CAD build for the part. Positions are in the model's coordinates, mm. Give positions to 0.01 mm unless a question says otherwise; leave off trailing zeros. Write each loop counter-clockwise with the first axis right and the second up, starting at its lowest first coordinate (ties: lowest second). Pieces come first, ordered by that corner, then holes. Notation, with made-up numbers: (-3.75, 54) -> (41.25, 54) arc R13 cw to (41.25, 71) -> close; hole circle Ø11 at (20.25, 67). An arc over 180 degrees is marked (long way). Answer in a Markdown table with one row per item. Add a question column.
```python
from build123d import *

# Parameters (mm, degrees)
SKETCH1_W           = 809.625
SKETCH1_H           = 555.625
SKETCH1_R           = 1.27
SKETCH1_W_2         = 136.525
SKETCH1_H_2         = 184.76057441
BOSS_EXTRUDE1_DEPTH = 4.318
CUT_EXTRUDE2_DEPTH  = 5.318


with BuildPart() as part:
    # Sketch1 → Boss-Extrude1 (new body, symmetric)
    with BuildSketch(Plane.XY):
        Rectangle(SKETCH1_W, SKETCH1_H)
        with Locations((319.0875, 265.1125)):
            Circle(SKETCH1_R, mode=Mode.SUBTRACT)
        with Locations((344.4875, 265.1125)):
            Circle(SKETCH1_R, mode=Mode.SUBTRACT)
        with Locations((369.8875, 265.1125)):
            Circle(SKETCH1_R, mode=Mode.SUBTRACT)
        with Locations((392.1125, 217.4875)):
            Circle(SKETCH1_R, mode=Mode.SUBTRACT)
        with Locations((392.1125, 242.8875)):
            Circle(SKETCH1_R, mode=Mode.SUBTRACT)
        with Locations((392.1125, 268.2875)):
            Circle(SKETCH1_R, mode=Mode.SUBTRACT)
        with Locations((-315.9125, -265.1125)):
            Circle(SKETCH1_R, mode=Mode.SUBTRACT)
        with Locations((-341.3125, -265.1125)):
            Circle(SKETCH1_R, mode=Mode.SUBTRACT)
        with Locations((-366.7125, -265.1125)):
            Circle(SKETCH1_R, mode=Mode.SUBTRACT)
        with Locations((-392.1125, -214.3125)):
            Circle(SKETCH1_R, mode=Mode.SUBTRACT)
        with Locations((-392.1125, -239.7125)):
            Circle(SKETCH1_R, mode=Mode.SUBTRACT)
        with Locations((-392.1125, -265.1125)):
            Circle(SKETCH1_R, mode=Mode.SUBTRACT)
        with Locations((-315.9125, 265.1125)):
            Circle(SKETCH1_R, mode=Mode.SUBTRACT)
        with Locations((-341.3125, 265.1125)):
            Circle(SKETCH1_R, mode=Mode.SUBTRACT)
        with Locations((-366.7125, 265.1125)):
            Circle(SKETCH1_R, mode=Mode.SUBTRACT)
        with Locations((-392.1125, 217.4875)):
            Circle(SKETCH1_R, mode=Mode.SUBTRACT)
        with Locations((-392.1125, 242.8875)):
            Circle(SKETCH1_R, mode=Mode.SUBTRACT)
        with Locations((-392.1125, 268.2875)):
            Circle(SKETCH1_R, mode=Mode.SUBTRACT)
        with Locations((319.0875, -265.1125)):
            Circle(SKETCH1_R, mode=Mode.SUBTRACT)
        with Locations((392.1125, -188.9125)):
            Circle(SKETCH1_R, mode=Mode.SUBTRACT)
        with Locations((392.1125, -214.3125)):
            Circle(SKETCH1_R, mode=Mode.SUBTRACT)
        with Locations((392.1125, -239.7125)):
            Circle(SKETCH1_R, mode=Mode.SUBTRACT)
        with Locations((392.1125, -265.1125)):
            Circle(SKETCH1_R, mode=Mode.SUBTRACT)
        with Locations((369.8875, -265.1125)):
            Circle(SKETCH1_R, mode=Mode.SUBTRACT)
        with Locations((344.4875, -265.1125)):
            Circle(SKETCH1_R, mode=Mode.SUBTRACT)
        with Locations((0, -185.432212795)):
            Rectangle(SKETCH1_W_2, SKETCH1_H_2)
    extrude(amount=BOSS_EXTRUDE1_DEPTH, both=True)

    # Sketch1<3> → Cut-Extrude2 (cut, symmetric)
    with BuildSketch(Plane.XY):
        Polygon((-308.956687333, -206.6798), (-308.956687333, -277.8125), (308.956687333, -277.8125), (308.956687333, -206.68615), (68.2625, -206.68615), (68.2625, -93.05192559), (-68.2625, -93.05192559), (-68.2625, -206.6798), align=None)
    cut_extrude2 = extrude(amount=CUT_EXTRUDE2_DEPTH, both=True, mode=Mode.SUBTRACT)

    # Mirror1: Cut-Extrude2 across plane
    add(cut_extrude2.mirror(Plane.ZX), mode=Mode.SUBTRACT)


solid = part.part
```
Item 1: Drop flat-ended pins along their axis: pin 1 Ø2 at (x, z) = (-67, -2.5) entering from -Y; pin 2 Ø4 at (x, y) = (319.09, -265.11) entering from -Z; pin 3 Ø3 at (x, z) = (248.5, 0.5) entering from +Y; pin 4 Ø1.5 at (x, y) = (392.11, -265.11) entering from +Z. Give the stop position or say it passes through.
Item 2: Slice it at B-B, the plane x = 218. List the corners of the cut face in (y, z), then the cut area to 3 significant figures.
Item 3: Probe L1, parallel to X at y = -238, z = -3.25; L2, parallel to X at y = -129, z = 0.25; L3, parallel to Y at x = -250, z = -3.75. List the from-to ranges inside material, lowest first. Write a range as from..to.
Item 4: Slice it at D-D, the plane x = -81.5. List the corners of the cut face in (y, z), then the cut area to 3 significant figures.
Item 5: Slice it at C-C, the plane z = 1.75. State how many separate pieces and enclosed holes the cut face has, then the cut area to 3 significant figures.
Item 6: Slice it at A-A, the plane y = -150. List the corners of the cut face in (x, z).
Answer key:
| question | item | result |
|---|---|---|
| 1 | pin 1 | stops at y = -93.05 |
| 1 | pin 2 | stops at z = -4.32 |
| 1 | pin 3 | stops at y = 206.69 |
| 1 | pin 4 | passes through |
| 2 | outline | (-206.69, -4.32) -> (206.69, -4.32) -> (206.69, 4.32) -> (-206.69, 4.32) -> close |
| 2 | area | 3,570 mm² |
| 3 | L1 | x = -404.81..-308.96, 308.96..404.81 |
| 3 | L2 | x = -404.81..-68.26, 68.26..404.81 |
| 3 | L3 | y = -206.68..206.68 |
| 4 | outline | (-206.68, -4.32) -> (206.68, -4.32) -> (206.68, 4.32) -> (-206.68, 4.32) -> close |
| 4 | area | 3,570 mm² |
| 5 | separate pieces | 1 |
| 5 | enclosed holes | 25 |
| 5 | area | 331,000 mm² |
| 6 | outline | (-404.81, -4.32) -> (-68.26, -4.32) -> (-68.26, 4.32) -> (-404.81, 4.32) -> close; (68.26, -4.32) -> (404.81, -4.32) -> (404.81, 4.32) -> (68.26, 4.32) -> close |
